```python
from build123d import *

# Parameters (mm, degrees)
F0_W     = 28
F0_H     = 50
F1_DEPTH = 5
F2_R     = 5
F3_DEPTH = 5
F4_R     = 14
F4_R_2   = 11
F5_DEPTH = 8
F6_R     = 1.5


with BuildPart() as f1:
    # F0 (on Top) → F1 (new body)
    with BuildSketch(Plane.XY):
        with Locations((14, 25)):
            Rectangle(F0_W, F0_H)
    extrude(amount=F1_DEPTH)

    # F2 (on face) → F3 (cut, through all)
    with BuildSketch(Plane.XY.offset(5)):
        with Locations((14, 25)):
            Circle(F2_R)
    extrude(amount=-F3_DEPTH, mode=Mode.SUBTRACT)

    # F4 (on face) → F5 (join)
    with BuildSketch(Plane.XY.offset(5)):
        with Locations((14, 25)):
            Circle(F4_R)
        with Locations((14, 25)):
            Circle(F4_R_2, mode=Mode.SUBTRACT)
    extrude(amount=F5_DEPTH)

    # F6
    f6_edges = [f1.edges().sort_by_distance(p)[0] for p in [
        (0, 25, 13),
    ]]
    fillet(f6_edges, radius=F6_R)


solid = f1.part
```
Geometry check sheet. Reference: the model listing, model coordinates, mm. A direction names the side the tool comes from. Coordinates: 2 decimals unless noted, no trailing zeros. Write each loop counter-clockwise with the first axis right and the second up, starting at its lowest first coordinate (ties: lowest second). Pieces come first, ordered by that corner, then holes. Notation, with made-up numbers: M -8.5,75 L 0.5,75 A13 cw 0.5,87 Z; hole C 48,72.25 d8. An arc over 180 degrees is marked long. Use one line per item in the form item = value. Start each with the question number.
1) Release check for a two-part mould opening along X. For faces 3 (the flat face through (14, 43, 5)), 4 (the flat face through (28, 25, 2)), 5 (the flat face through (0, 25, 2)), 6 (the flat face through (19, 23, 5)) record: pulls with the +X half, pulls with the -X half, needs draft (parallel to the pull), parting line crosses it, or undercut.
2) Go/stop test with flat-tipped pins: pin 1 Ø9 at (x, y) = (14, 25) entering from -Z; pin 2 Ø1 at (x, z) = (9.5, 11.5) entering from +Y; pin 3 Ø7.5 at (x, y) = (9, 6.5) entering from +Z; pin 4 Ø12.5 at (x, y) = (9, 43.5) entering from +Z. Record where each tip stops, or that it passes through.
3) Thickness scan on probe 1 along Y at (x, z) = (14, 3.2); probe 2 along Y at (x, z) = (14, 7.25); probe 3 along Z at (x, y) = (24, 7.5). Record the ranges inside material, lowest first. Write a range as from..to.
4) Section check A-A on x = 14. Enter the section's corners in (y, z), and give its area (3 significant figures).
5) Section check B-B on z = 1.75. Enter the section's corners in (x, y).
6) Set-up check for faces 1 (the flat face through (14, 0, 2)), 2 (the cylindrical face through (11.62, 14.26, 8.94)): record each of +Z, -Z, +X, -X, +Y, -Y from which the full face is reachable in a straight line by a thin tool's end or side.
Responses:
q1.face_3 = needs draft
q1.face_4 = pulls with the +X half
q1.face_5 = pulls with the -X half
q1.face_6 = undercut
q2.pin_1 = through
q2.pin_2 = 38.42
q2.pin_3 = 5
q2.pin_4 = 12.94
q3.probe_1 = 0..20, 30..50
q3.probe_2 = 11..14, 36..39
q3.probe_3 = 0..5
q4.outline = M 0,0 L 20,0 L 20,5 L 14,5 L 14,13 L 12.5,13 A1.5 ccw 11,11.5 L 11,5 L 0,5 Z; M 30,0 L 50,0 L 50,5 L 39,5 L 39,11.5 A1.5 ccw 37.5,13 L 36,13 L 36,5 L 30,5 Z
q4.area = 247 mm2
q5.outline = M 0,0 L 28,0 L 28,50 L 0,50 Z; hole C 14,25 d10
q6.face_1 = +Z, -Z, +X, -X, -Y
q6.face_2 = +Z
